Can you work these out from the model? Positions are in its coordinate system, mm. A direction names the side the tool comes from. Coordinates: 2 decimals unless noted, no trailing zeros. Order: outer loops, then holes, each group sorted by start corner. A loop starts at its lowest first (then second) coordinate and runs counter-clockwise, first axis right, second up.
```python
from build123d import *

# Parameters (mm, degrees)
ESQUISSE1_R        = 1.5
BOSS_EXTRU_2_DEPTH = 6


with BuildPart() as part:
    # Esquisse1 → Boss.-Extru.2 (new body)
    with BuildSketch(Plane.XY):
        with BuildLine():
            Line((-6, -33.155494421), (-6, -30.155494421))
            Line((-6, -30.155494421), (-7, -30.155494421))
            Line((-7, -30.155494421), (-7, -26.155494421))
            Line((-7, -26.155494421), (-6, -26.155494421))
            Line((-6, -26.155494421), (-6, -19.805494421))
            Line((-6, -19.805494421), (6, -19.805494421))
            Line((6, -19.805494421), (6, -26.155494421))
            Line((6, -26.155494421), (7, -26.155494421))
            Line((7, -26.155494421), (7, -30.155494421))
            Line((7, -30.155494421), (6, -30.155494421))
            Line((6, -30.155494421), (6, -33.155494421))
            Line((6, -33.155494421), (10, -33.155494421))
            Line((10, -33.155494421), (10, -16.155494421))
            ThreePointArc((10, -16.155494421), (0, 19), (-10, -16.155494421))
            Line((-10, -16.155494421), (-10, -33.155494421))
            Line((-10, -33.155494421), (-6, -33.155494421))
        make_face()
        with Locations((0, 14)):
            Circle(ESQUISSE1_R, mode=Mode.SUBTRACT)
        with Locations((12.124355653, -7)):
            Circle(ESQUISSE1_R, mode=Mode.SUBTRACT)
        with Locations((-12.124355653, -7)):
            Circle(ESQUISSE1_R, mode=Mode.SUBTRACT)
        with BuildLine():
            Line((6, -16.805494421), (-6, -16.805494421))
            Line((-6, -16.805494421), (-6, -12.649110641))
            ThreePointArc((-6, -12.649110641), (-6.653410863, -12.317959405), (-7.288606081, -11.953084179))
            ThreePointArc((-7.288606081, -11.953084179), (-8.912631465, -10.307392628), (-9.031496673, -7.998360322))
            ThreePointArc((-9.031496673, -7.998360322), (-9.309773091, -5.375), (-11.442531564, -3.822325392))
            ThreePointArc((-11.442531564, -3.822325392), (-13.054716827, -2.946828253), (-13.935938611, -1.337764944))
            ThreePointArc((-13.935938611, -1.337764944), (-12.367555464, 6.560760004), (-6.707371512, 12.288660114))
            ThreePointArc((-6.707371512, 12.288660114), (-4.47014813, 12.872261577), (-2.411034891, 11.820685714))
            ThreePointArc((-2.411034891, 11.820685714), (0, 10.75), (2.411034891, 11.820685714))
            ThreePointArc((2.411034891, 11.820685714), (3.975330286, 12.779130538), (5.80943088, 12.737759334))
            ThreePointArc((5.80943088, 12.737759334), (11.865562564, 7.430237213), (13.995977593, -0.335575935))
            ThreePointArc((13.995977593, -0.335575935), (13.382779595, -2.564868949), (11.442531564, -3.822325392))
            ThreePointArc((11.442531564, -3.822325392), (9.309773091, -5.375), (9.031496673, -7.998360322))
            ThreePointArc((9.031496673, -7.998360322), (9.079386541, -9.832302285), (8.126507731, -11.399994391))
            ThreePointArc((8.126507731, -11.399994391), (7.090812931, -12.071469338), (6, -12.649110641))
            Line((6, -12.649110641), (6, -16.805494421))
        make_face(mode=Mode.SUBTRACT)
    extrude(amount=BOSS_EXTRU_2_DEPTH)


solid = part.part
```
1. Please list where these lines run through material, in increasing order: probe 1 along Y at (x, z) = (0, 2.35); probe 2 along X at (y, z) = (-6, 3.5); probe 3 along Y at (x, z) = (-11, 4.65).
Completed:
probe 1: y = -19.81 to -16.81, 10.75 to 12.5, 15.5 to 19
probe 2: x = -18.03 to -13.24, -11.01 to -9.03, 9.03 to 11.01, 13.24 to 18.03
probe 3: y = -15.49 to -7.99, -6.01 to -3.95, 8.66 to 15.49
2. I'm going to push flat-ended pins straight in: pin 1 (3.5 mm diameter, centred on y = -31, z = 3.5, fed in from +X); pin 2 (3 mm diameter, centred on x = 4, z = 2, fed in from -Y); pin 3 (1.5 mm diameter, centred on y = -4.5, z = 3.5, fed in from -X). Where does each tip first touch, or does it pass through?
Completed:
pin 1: stops at x = 10
pin 2: stops at y = -19.81
pin 3: stops at x = -18.63
3. Imagine slicing it at D-D on x = 12. Please give me the cut outline in (y, z).
Completed:
outline: (-14.73, 0) - (-8.49, 0) - (-8.49, 6) - (-14.73, 6) - close; (-5.51, 0) - (-3.65, 0) - (-3.65, 6) - (-5.51, 6) - close; (7.21, 0) - (14.73, 0) - (14.73, 6) - (7.21, 6) - close
4. Thinking about a two-plate mould opening in X: for faces 1 (the flat face through (-10, -25, 3)), 2 (the flat face through (-10, -5, 6)), 3 (the flat face through (0, -16.805, 3)), which applies, pulls with the +X half, pulls with the -X half, needs draft (parallel to the pull), parting line crosses it, or undercut?
Completed:
face 1: pulls with the -X half
face 2: needs draft
face 3: undercut
5. Imagine slicing it at C-C on y = -7. Please give me the cut outline in (x, z), then the cut area to 3 significant figures.
Completed:
outline: (-17.66, 0) - (-13.62, 0) - (-13.62, 6) - (-17.66, 6) - close; (-10.62, 0) - (-8.87, 0) - (-8.87, 6) - (-10.62, 6) - close; (8.87, 0) - (10.62, 0) - (10.62, 6) - (8.87, 6) - close; (13.62, 0) - (17.66, 0) - (17.66, 6) - (13.62, 6) - close
area: 69.5 mm2
6. On a 3-axis mill with a long thin cutter (end or side, diameter ignored), from which of +Z, -Z, +X, -X, +Y, -Y can I reach the whole of each face in a straight line? I mean faces 4 (the flat face through (-6, -32, 3)), 5 (the flat face through (-8, -33.155, 3)), 6 (the flat face through (-6.5, -30.155, 3)). Say none if no direction works.
Completed:
face 4: +Z, -Z, -Y
face 5: +Z, -Z, +X, -X, -Y
face 6: +Z, -Z
7. Imagine slicing it at B-B on y = 2.5. Please give me the cut outline in (x, z).
Completed:
outline: (-18.83, 0) - (-13.77, 0) - (-13.77, 6) - (-18.83, 6) - close; (13.77, 0) - (18.83, 0) - (18.83, 6) - (13.77, 6) - close
8. Imagine slicing it at A-A on x = 0. Please give me the cut outline in (y, z).
Completed:
outline: (-19.81, 0) - (-16.81, 0) - (-16.81, 6) - (-19.81, 6) - close; (10.75, 0) - (12.5, 0) - (12.5, 6) - (10.75, 6) - close; (15.5, 0) - (19, 0) - (19, 6) - (15.5, 6) - close
